Here's how the part is built. I have some questions about the finished solid (model axes, mm). Round coordinates to 2 decimals unless told otherwise and drop trailing zeros. Write each loop counter-clockwise with the first axis right and the second up, starting at its lowest first coordinate (ties: lowest second). Pieces come first, ordered by that corner, then holes. Notation, with made-up numbers: M 28.25,55.25 L 41.25,55.25 A8 cw 41.25,68.25 Z; hole C -14.5,85.5 d5. An arc over 180 degrees is marked long. Use a Markdown table: item, result. Add a question column.
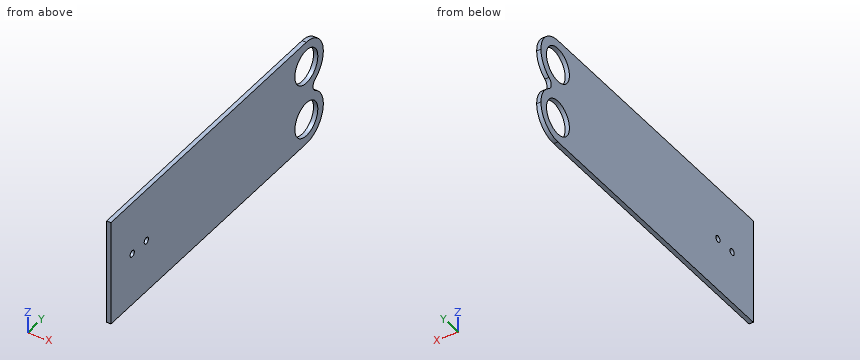
```python
from build123d import *

# Parameters (mm, degrees)
SKETCH1_W               = 2
SKETCH1_H               = 150
BOSS_EXTRUDE1_DEPTH     = 50
SKETCH3_R               = 8.1
CUT_EXTRUDE2_DEPTH      = 50
SKETCH4_R               = 1.5
CUT_EXTRUDE3_DEPTH      = 1
CUT_EXTRUDE3_DEPTH_BACK = 3


with BuildPart() as part:
    # Sketch1 → Boss-Extrude1 (new body)
    with BuildSketch(Plane.XY):
        with Locations((1, -40)):
            Rectangle(SKETCH1_W, SKETCH1_H)
    extrude(amount=BOSS_EXTRUDE1_DEPTH)

    # Sketch3 → Cut-Extrude2 (cut)
    with BuildSketch(Plane(origin=(2, 0, 0), x_dir=(0, 0, -1), z_dir=(1, 0, 0))):
        with Locations((-12, 23)):
            Circle(SKETCH3_R)
        with Locations((-38, 23)):
            Circle(SKETCH3_R)
        with BuildLine():
            ThreePointArc((-50, 23), (-46.485281374, 31.485281374), (-38, 35))
            Line((-38, 35), (-50, 35))
            Line((-50, 35), (-50, 23))
        make_face()
        with BuildLine():
            ThreePointArc((-22.2198998, 29.289169108), (-17.8536301, 33.475448184), (-12, 35))
            Line((-12, 35), (-38, 35))
            ThreePointArc((-38, 35), (-32.1463699, 33.475448184), (-27.7801002, 29.289169108))
            ThreePointArc((-27.7801002, 29.289169108), (-25, 27.735662478), (-22.2198998, 29.289169108))
        make_face()
        with BuildLine():
            Line((0, 35), (-12, 35))
            ThreePointArc((-12, 35), (-3.514718626, 31.485281374), (0, 23))
            Line((0, 23), (0, 35))
        make_face()
    extrude(amount=-CUT_EXTRUDE2_DEPTH, mode=Mode.SUBTRACT)

    # Sketch4 → Cut-Extrude3 (cut, two sides)
    with BuildSketch(Plane.ZY) as cut_extrude3_sk:
        with Locations((25, -100)):
            Circle(SKETCH4_R)
        with Locations((25, -90)):
            Circle(SKETCH4_R)
    extrude(amount=CUT_EXTRUDE3_DEPTH, mode=Mode.SUBTRACT)
    extrude(cut_extrude3_sk.sketch, amount=-CUT_EXTRUDE3_DEPTH_BACK, mode=Mode.SUBTRACT)


solid = part.part
```
Item 1: Imagine slicing it at A-A on y = -90. List the corners of the cut face in (x, z) for me.
Item 2: Imagine slicing it at C-C on y = 25.5. List the corners of the cut face in (x, z) for me, plus the area to 3 significant figures.
Item 3: Imagine slicing it at B-B on z = 25. List the corners of the cut face in (x, y) for me, plus the area to 3 significant figures.
Item 4: For pin 1 Ø1.8 at (y, z) = (-100, 25) entering from +X, with a flat end and sliding along its axis, tell me the tip position at first contact or that it passes through.
Item 5: I need wall thicknesses on probe 1 along Z at (x, y) = (1.4, -90); probe 2 along Y at (x, z) = (1.2, 12); probe 3 along Y at (x, z) = (1.3, 25). Which ranges of each line are inside material? Lowest first, please. Write a range as from..to.
Item 6: Imagine slicing it at D-D on z = 40. List the corners of the cut face in (x, y) for me.
The answers:
| question | item | result |
|---|---|---|
| 1 | outline | M 0,0 L 2,0 L 2,23.5 L 0,23.5 Z; M 0,26.5 L 2,26.5 L 2,50 L 0,50 Z |
| 2 | outline | M 0,0.26 L 2,0.26 L 2,4.3 L 0,4.3 Z; M 0,19.7 L 2,19.7 L 2,30.3 L 0,30.3 Z; M 0,45.7 L 2,45.7 L 2,49.74 L 0,49.74 Z |
| 2 | area | 37.3 mm² |
| 3 | outline | M 0,-115 L 2,-115 L 2,-101.5 L 0,-101.5 Z; M 0,-98.5 L 2,-98.5 L 2,-91.5 L 0,-91.5 Z; M 0,-88.5 L 2,-88.5 L 2,27.74 L 0,27.74 Z |
| 3 | area | 273 mm² |
| 4 | pin 1 | through |
| 5 | probe 1 | 0..23.5, 26.5..50 |
| 5 | probe 2 | -115..14.9, 31.1..35 |
| 5 | probe 3 | -115..-101.5, -98.5..-91.5, -88.5..27.74 |
| 6 | outline | M 0,-115 L 2,-115 L 2,15.15 L 0,15.15 Z; M 0,30.85 L 2,30.85 L 2,34.83 L 0,34.83 Z |
